The model under review builds one solid part; all positions refer to its coordinate system, in mm. Coordinates: 2 decimals unless noted, no trailing zeros. Loops run counter-clockwise (first coordinate to the right, second up) from the corner with the lowest first, then second, coordinate; pieces in that order, holes last. Notation, with made-up numbers: M -24.75,53.25 L 26.25,53.25 A16 cw 26.25,77.25 Z; hole C -18.75,-16 d6. An arc over 180 degrees is marked long. One line per item, written item: value.
```python
from build123d import *

# Parameters (mm, degrees)
F0_W     = 1219.2
F0_H     = 2133.6
F1_DEPTH = 609.6
F2_W     = 1168.4
F2_H     = 381
F3_DEPTH = 609.601
F4_W     = 558.8
F4_H     = 381
F5_DEPTH = 1219.201


with BuildPart() as f1:
    # F0 (on Front) → F1 (new body)
    with BuildSketch(Plane.XZ):
        Rectangle(F0_W, F0_H)
    extrude(amount=F1_DEPTH)

    # F2 (on face) → F3 (cut, through all)
    with BuildSketch(Plane.XZ.offset(609.6)):
        with Locations((0, 850.9)):
            Rectangle(F2_W, F2_H)
        with Locations((0, 424.18)):
            Rectangle(F2_W, F2_H)
        with Locations((0, -2.54)):
            Rectangle(F2_W, F2_H)
        with Locations((0, -429.26)):
            Rectangle(F2_W, F2_H)
        with Locations((0, -855.98)):
            Rectangle(F2_W, F2_H)
    extrude(amount=-F3_DEPTH, mode=Mode.SUBTRACT)

    # F4 (on face) → F5 (cut, through all)
    with BuildSketch(Plane(origin=(-609.6, 0, 0), x_dir=(0, -1, 0), z_dir=(-1, 0, 0))):
        with Locations((304.8, 850.9)):
            Rectangle(F4_W, F4_H)
        with Locations((304.8, 424.18)):
            Rectangle(F4_W, F4_H)
        with Locations((304.8, -2.54)):
            Rectangle(F4_W, F4_H)
        with Locations((304.8, -429.26)):
            Rectangle(F4_W, F4_H)
        with Locations((304.8, -855.98)):
            Rectangle(F4_W, F4_H)
    extrude(amount=-F5_DEPTH, mode=Mode.SUBTRACT)


solid = f1.part
```
(1) To check wall thickness, follow L1, parallel to Z at x = -50, y = -142. State the ranges of the line that lie inside material, in increasing order. Write a range as [from, to].
Checks:
L1: [-1066.8, -1046.48], [-665.48, -619.76], [-238.76, -193.04], [187.96, 233.68], [614.68, 660.4], [1041.4, 1066.8]
(2) Insertion check: pin 1 Ø20.5 at (x, z) = (591.5, 81.5) entering from +Y. The pin has a flat end and moves straight along its axis. Give the tip position at first contact, or say it passes through.
Checks:
pin 1: y = 0
(3) Draft analysis for pull direction Z (two halves, no side actions). For faces 1 (the face through (-9, -301, 614.68)), 2 (the face through (-9, -301, 1066.8)), 3 (the face through (-183, 0, -232)), 4 (the face through (-9, -301, -1066.8)), state which applies: pulls with the +Z half, pulls with the -Z half, needs draft (parallel to the pull), parting line crosses it, or undercut.
Checks:
face 1: undercut
face 2: pulls with the +Z half
face 3: needs draft
face 4: pulls with the -Z half
(4) Add section C-C on y = -393. State the section outline as (x, z) points.
Checks:
outline: M -609.6,-1066.8 L 609.6,-1066.8 L 609.6,-1046.48 L -609.6,-1046.48 Z; M -609.6,-665.48 L 609.6,-665.48 L 609.6,-619.76 L -609.6,-619.76 Z; M -609.6,-238.76 L 609.6,-238.76 L 609.6,-193.04 L -609.6,-193.04 Z; M -609.6,187.96 L 609.6,187.96 L 609.6,233.68 L -609.6,233.68 Z; M -609.6,614.68 L 609.6,614.68 L 609.6,660.4 L -609.6,660.4 Z; M -609.6,1041.4 L 609.6,1041.4 L 609.6,1066.8 L -609.6,1066.8 Z
(5) Add section A-A on z = -710. State the section outline as (x, y) points, then the cut area to 3 significant figures.
Checks:
outline: M -609.6,-609.6 L -584.2,-609.6 L -584.2,-584.2 L -609.6,-584.2 Z; M -609.6,-25.4 L -584.2,-25.4 L -584.2,0 L -609.6,0 Z; M 584.2,-609.6 L 609.6,-609.6 L 609.6,-584.2 L 584.2,-584.2 Z; M 584.2,-25.4 L 609.6,-25.4 L 609.6,0 L 584.2,0 Z
area: 2,580 mm^2
(6) Add section B-B on x = 53.5. State the section outline as (y, z) points.
Checks:
outline: M -609.6,-1066.8 L 0,-1066.8 L 0,-1046.48 L -609.6,-1046.48 Z; M -609.6,-665.48 L 0,-665.48 L 0,-619.76 L -609.6,-619.76 Z; M -609.6,-238.76 L 0,-238.76 L 0,-193.04 L -609.6,-193.04 Z; M -609.6,187.96 L 0,187.96 L 0,233.68 L -609.6,233.68 Z; M -609.6,614.68 L 0,614.68 L 0,660.4 L -609.6,660.4 Z; M -609.6,1041.4 L 0,1041.4 L 0,1066.8 L -609.6,1066.8 Z
